from build123d import *

# Parameters (mm, degrees)
SKETCH001_R     = 25
PAD_DEPTH       = 0.5
PAD001_DEPTH    = 5
SKETCH002_R     = 2.5
PAD002_DEPTH    = 10
SKETCH003_R     = 4
SKETCH003_R_2   = 3
PAD003_DEPTH    = 20
SKETCH004_R     = 3
POCKET_DEPTH    = 20.501
CHAMFER_SIZE    = 1
CHAMFER001_SIZE = 0.5


with BuildPart() as part:
    # Sketch001 → Pad (new body)
    with BuildSketch(Plane.XY):
        Circle(SKETCH001_R)
    extrude(amount=PAD_DEPTH)

    # Sketch → Pad001 (join)
    with BuildSketch(Plane.XY):
        Polygon((0, 24), (-3.897114, 21.75), (-3.897114, 17.25), (0, 15), (3.897114, 17.25), (3.897114, 21.75), align=None)
        Polygon((16.606239, -5.258798), (12.857372, -7.747974), (13.138629, -12.239176), (17.168752, -14.241202), (20.917619, -11.752026), (20.636362, -7.260824), align=None)
        Polygon((-18.222418, -5.452561), (-21.276648, -8.757357), (-19.941725, -13.054796), (-15.552573, -14.047439), (-12.498343, -10.742643), (-13.833265, -6.445204), align=None)
    extrude(amount=PAD001_DEPTH)

    # Sketch002 (on Face25 of Pad001) → Pad002 (join)
    with BuildSketch(Plane.XY.offset(5)):
        with Locations((0, 19.5)):
            Circle(SKETCH002_R)
        with Locations((16.887495, -9.75)):
            Circle(SKETCH002_R)
        with Locations((-16.887495, -9.75)):
            Circle(SKETCH002_R)
    extrude(amount=PAD002_DEPTH)

    # Sketch003 (on Face3 of Pad002) → Pad003 (join)
    with BuildSketch(Plane.XY.offset(0.5)):
        Circle(SKETCH003_R)
        Circle(SKETCH003_R_2, mode=Mode.SUBTRACT)
    extrude(amount=PAD003_DEPTH)

    # Sketch004 (on Face2 of Pad003) → Pocket (cut, through all)
    with BuildSketch(Plane(origin=(0, 0, 0), x_dir=(1, 0, 0), z_dir=(0, 0, -1))):
        Circle(SKETCH004_R)
    extrude(amount=-POCKET_DEPTH, mode=Mode.SUBTRACT)

    # Chamfer
    chamfer_edges = [part.edges().sort_by_distance(p)[0] for p in [
        (-19.387495, -9.75, 15),
        (-2.5, 19.5, 15),
        (14.387495, -9.75, 15),
    ]]
    chamfer(chamfer_edges, length=CHAMFER_SIZE)

    # Chamfer001
    chamfer001_edges = [part.edges().sort_by_distance(p)[0] for p in [
        (-4, 0, 20.5),
    ]]
    chamfer(chamfer001_edges, length=CHAMFER001_SIZE)


solid = part.part
CAD build for the part. Positions are in the model's coordinates, mm. A direction names the side the tool comes from. Give positions to 0.01 mm unless a question says otherwise; leave off trailing zeros. Order: outer loops, then holes, each group sorted by start corner. A loop starts at its lowest first (then second) coordinate and runs counter-clockwise, first axis right, second up. Notation, with made-up numbers: (18.25, 57) -> (42.25, 57) arc R17 ccw to (42.25, 79) -> close; hole circle Ø8 at (86.5, 61.5). An arc over 180 degrees is marked (long way). Return JSON: item names as keys, results as strings.
Q1. Saw through at A-A (z = 2). Write the cut outline in (x, y).
Working result:
{"outline": "(-21.28, -8.76) -> (-19.94, -13.05) -> (-15.55, -14.05) -> (-12.5, -10.74) -> (-13.83, -6.45) -> (-18.22, -5.45) -> close; circle Ø8 at (0, 0); (-3.9, 17.25) -> (0, 15) -> (3.9, 17.25) -> (3.9, 21.75) -> (0, 24) -> (-3.9, 21.75) -> close; (12.86, -7.75) -> (13.14, -12.24) -> (17.17, -14.24) -> (20.92, -11.75) -> (20.64, -7.26) -> (16.61, -5.26) -> close; hole circle Ø6 at (0, 0)"}
Q2. Saw through at C-C (z = 6). Write the cut outline in (x, y).
Working result:
{"outline": "circle Ø5 at (-16.89, -9.75); circle Ø8 at (0, 0); circle Ø5 at (0, 19.5); circle Ø5 at (16.89, -9.75); hole circle Ø6 at (0, 0)"}
Q3. Flat gauge pins, fed straight in: pin 1 (2.5 mm diameter, centred on x = 0.5, y = 21.5, fed in from +Z); pin 2 (6 mm diameter, centred on x = 2.5, z = 13.5, fed in from +Y); pin 3 (25 mm diameter, centred on x = 5.5, y = -2.5, fed in from +Z); pin 4 (1.5 mm diameter, centred on x = -13.5, z = 14.5, fed in from -Y). Where does each tip first touch, or does it go through?
Working result:
{"pin 1": "z = 15", "pin 2": "y = 22", "pin 3": "z = 20.5", "pin 4": "through"}
Q4. Mould opens along Y. For faces 1 (the face through (3, 20, 5)), 2 (the face through (14.904, -11.271, 9.437)), 3 (the face through (-1.976, 16.141, 2.718)), 4 (the face through (-19, -12, 5)) say: pulls with the +Y half, pulls with the -Y half, needs draft (parallel to the pull), parting line crosses it, or undercut.
Working result:
{"face 1": "undercut", "face 2": "parting line crosses it", "face 3": "undercut", "face 4": "needs draft"}
Q5. Saw through at B-B (y = 0). Write the cut outline in (x, z), then the cut area to 4 significant figures.
Working result:
{"outline": "(-25, 0) -> (-3, 0) -> (-3, 20.5) -> (-3.5, 20.5) -> (-4, 20) -> (-4, 0.5) -> (-25, 0.5) -> close; (3, 0) -> (25, 0) -> (25, 0.5) -> (4, 0.5) -> (4, 20) -> (3.5, 20.5) -> (3, 20.5) -> close", "area": "61.75 mm²"}
Q6. Saw through at D-D (y = 19.5). Write the cut outline in (x, z).
Working result:
{"outline": "(-15.64, 0) -> (15.64, 0) -> (15.64, 0.5) -> (3.9, 0.5) -> (3.9, 5) -> (2.5, 5) -> (2.5, 14) -> (1.5, 15) -> (-1.5, 15) -> (-2.5, 14) -> (-2.5, 5) -> (-3.9, 5) -> (-3.9, 0.5) -> (-15.64, 0.5) -> close"}
Q7. Drill centre lines: line 1 (Y direction, x = 0, z = 6.75); line 2 (Y direction, x = 0, z = 16); line 3 (X direction, y = 1, z = 13.75). Where is each one in solid material? Low to high.
Working result:
{"line 1": "-4 to -3, 3 to 4, 17 to 22", "line 2": "-4 to -3, 3 to 4", "line 3": "-3.87 to -2.83, 2.83 to 3.87"}
Q8. Which spindle directions (+Z, -Z, +X, -X, +Y, -Y) get a long thin tool onto all of the face, cutting with end or side? Do faces 5 (the face through (-13.156, -8.624, 2.718)), 6 (the face through (-15.734, -11.968, 9.437)), 7 (the face through (19.02, -13.01, 2.72)), 8 (the face through (-17.778, -13.544, 2.718)). Say none if no direction does.
Working result:
{"face 5": "+Z, +Y", "face 6": "+Z", "face 7": "+Z, +X, -Y", "face 8": "+Z, -X, -Y"}
